Check sheet for the modelled part. Datum: model origin and axes. Units: mm. Face numbers are marked on the shaded views. A direction names the side the tool comes from. Coordinates: 2 decimals unless noted, no trailing zeros. Write each loop counter-clockwise with the first axis right and the second up, starting at its lowest first coordinate (ties: lowest second). Pieces come first, ordered by that corner, then holes. Notation, with made-up numbers: (62.5, -38.5) -> (111.5, -38.5) arc R23 cw to (111.5, -11.5) -> close; hole circle Ø1 at (78.25, 86). An arc over 180 degrees is marked (long way). Put each result on its own line as item: value.
```python
from build123d import *

# Parameters (mm, degrees)
F0_W      = 63.5
F0_H      = 47.625
F1_DEPTH  = 76.2
F2_W      = 41.275
F2_H      = 63.5
F3_DEPTH  = 25.4
F4_R      = 8.255
F6_W      = 12.7
F6_H      = 15.875
F7_DEPTH  = 1.5875
F8_R      = 3.175
F9_W      = 3.175
F9_H      = 6.35
F10_DEPTH = 25.4
F11_R     = 1.58749
F12_W     = 25.4
F12_H     = 47.625
F13_DEPTH = 1.5875
F14_R     = 1.5875


# Not quite as in the source:
# - a fillet or chamfer is up to 0.001 mm smaller than in the source, because OpenCascade refuses the exact size


with BuildPart() as f1:
    # F0 (on Top) → F1 (new body)
    with BuildSketch(Plane.XY):
        Rectangle(F0_W, F0_H)
    extrude(amount=F1_DEPTH)

    # F2 (on face) → F3 (join)
    with BuildSketch(Plane.XZ.offset(23.8125)):
        with Locations((0, 33.3375)):
            Rectangle(F2_W, F2_H)
    extrude(amount=F3_DEPTH)

    # F4
    f4_edges = [f1.edges().sort_by_distance(p)[0] for p in [
        (-20.6375, -36.5125, 65.0875),
        (20.6375, -36.5125, 65.0875),
        (-20.6375, -36.5125, 1.5875),
        (20.6375, -36.5125, 1.5875),
        (20.6375, -49.2125, 33.3375),
        (0, -49.2125, 65.0875),
        (-20.6375, -49.2125, 33.3375),
        (0, -49.2125, 1.5875),
    ]]
    fillet(f4_edges, radius=F4_R)

    # F5: F1 across plane


with BuildPart() as f1_1:
    add(f1.part)
    add(f1.part.mirror(Plane.XZ))

    # F6 (on face) → F7 (join)
    with BuildSketch(Plane(origin=(0, 0, 0), x_dir=(1, 0, 0), z_dir=(0, 0, -1))):
        with Locations((-25.4, 31.75)):
            Rectangle(F6_W, F6_H)
        with Locations((25.4, 31.75)):
            Rectangle(F6_W, F6_H)
        with Locations((25.4, -31.75)):
            Rectangle(F6_W, F6_H)
        with Locations((-25.4, -31.75)):
            Rectangle(F6_W, F6_H)
    extrude(amount=-F7_DEPTH)

    # F8
    f8_edges = [f1_1.edges().sort_by_distance(p)[0] for p in [
        (-31.75, -39.6875, 0.79375),
        (-19.05, -39.6875, 0.79375),
        (19.05, -39.6875, 0.79375),
        (31.75, -39.6875, 0.79375),
        (31.75, 39.6875, 0.79375),
        (19.05, 39.6875, 0.79375),
        (-19.05, 39.6875, 0.79375),
        (-31.75, 39.6875, 0.79375),
    ]]
    fillet(f8_edges, radius=F8_R)

    # F9 (on face) → F10 (cut)
    with BuildSketch(Plane(origin=(0, 0, 0), x_dir=(1, 0, 0), z_dir=(0, 0, -1))):
        with Locations((-25.4, 31.75)):
            Rectangle(F9_W, F9_H)
        with Locations((25.4, 31.75)):
            Rectangle(F9_W, F9_H)
        with Locations((25.4, -31.75)):
            Rectangle(F9_W, F9_H)
        with Locations((-25.4, -31.75)):
            Rectangle(F9_W, F9_H)
    extrude(amount=-F10_DEPTH, mode=Mode.SUBTRACT)

    # F11 (radius 1.5875 in the source; OpenCascade refuses exactly that, so slightly less here)
    f11_edges = [f1_1.edges().sort_by_distance(p)[0] for p in [
        (-26.9875, -34.925, 0.79375),
        (-23.8125, -34.925, 0.79375),
        (-26.9875, -28.575, 0.79375),
        (-23.8125, -28.575, 0.79375),
        (26.9875, -28.575, 0.79375),
        (26.9875, -34.925, 0.79375),
        (23.8125, -34.925, 0.79375),
        (23.8125, -28.575, 0.79375),
        (-26.9875, 34.925, 0.79375),
        (-23.8125, 34.925, 0.79375),
        (-23.8125, 28.575, 0.79375),
        (-26.9875, 28.575, 0.79375),
        (23.8125, 28.575, 0.79375),
        (26.9875, 34.925, 0.79375),
        (23.8125, 34.925, 0.79375),
        (26.9875, 28.575, 0.79375),
    ]]
    fillet(f11_edges, radius=F11_R)

    # F12 (on face) → F13 (join)
    with BuildSketch(Plane.XY.offset(76.2)):
        Rectangle(F12_W, F12_H)
    extrude(amount=F13_DEPTH)

    # F14
    f14_edges = [f1_1.edges().sort_by_distance(p)[0] for p in [
        (0, -23.8125, 77.7875),
        (0, 23.8125, 77.7875),
    ]]
    fillet(f14_edges, radius=F14_R)


solid = f1_1.part
```
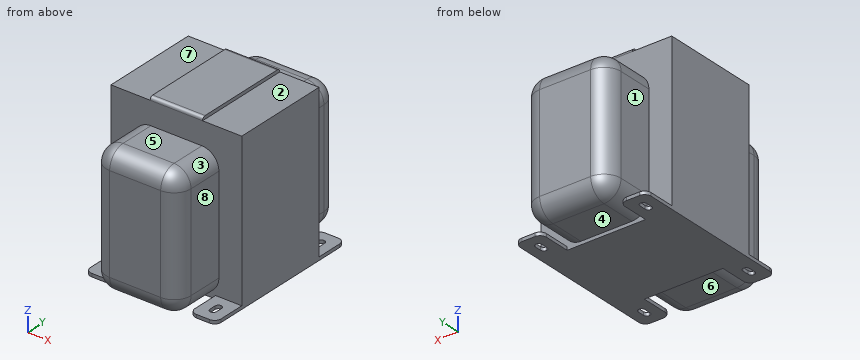
Q1. Material ranges on line 1 along X through (y, z) = (34.5, 10); line 2 along Z through (x, y) = (23.5, 14.5); line 3 along Z through (x, y) = (-21.5, -39), recorded low to high.
Recorded:
line 1: x = -20.64 to 20.64
line 2: z = 0 to 76.2
line 3: z = 0 to 1.59
Q2. Cross-section at A-A (x = 0). Record the cut outline in (y, z) (1 decimal).
Recorded:
outline: (-49.2, 9.8) arc R8.3 ccw to (-41, 1.6) -> (-23.8, 1.6) -> (-23.8, 0) -> (23.8, 0) -> (23.8, 1.6) -> (41, 1.6) arc R8.3 ccw to (49.2, 9.8) -> (49.2, 56.8) arc R8.3 ccw to (41, 65.1) -> (23.8, 65.1) -> (23.8, 76.2) arc R1.6 ccw to (22.2, 77.8) -> (-22.2, 77.8) arc R1.6 ccw to (-23.8, 76.2) -> (-23.8, 65.1) -> (-41, 65.1) arc R8.3 ccw to (-49.2, 56.8) -> close
Q3. Mould release check, pull along X, two halves, no side actions. Record for the marked faces 6, 7 and 8: released by +X, released by -X, zero draft, split by the parting line, or undercut.
Recorded:
face 6: undercut
face 7: zero draft
face 8: released by +X
Q4. Cross-section at D-D (z = 67.5). Record the cut outline in (x, y), plus the area to 3 significant figures.
Recorded:
outline: (-31.75, -23.81) -> (31.75, -23.81) -> (31.75, 23.81) -> (-31.75, 23.81) -> close
area: 3,020 mm2
Q5. Cross-section at C-C (z = 59). Record the cut outline in (x, y).
Recorded:
outline: (-31.75, -23.81) -> (-20.35, -23.81) -> (-20.35, -40.96) arc R7.97 ccw to (-12.38, -48.92) -> (12.38, -48.92) arc R7.97 ccw to (20.35, -40.96) -> (20.35, -23.81) -> (31.75, -23.81) -> (31.75, 23.81) -> (20.35, 23.81) -> (20.35, 40.96) arc R7.97 ccw to (12.38, 48.92) -> (-12.38, 48.92) arc R7.97 ccw to (-20.35, 40.96) -> (-20.35, 23.81) -> (-31.75, 23.81) -> close
Q6. Depth check by flat-ended pin: P1, Ø1.3, axis at y = 2.5, z = 77, coming from the -X side; P2, Ø0.8, axis at x = 25, z = 1, coming from the -Y side; P3, Ø6, axis at x = -24, y = 11.5, coming from the +Z side. Enter the tip coordinate at first touch or a pass-through.
Recorded:
P1: stops at x = -12.7
P2: stops at y = -39.69
P3: stops at z = 76.2
Q7. Tool access check on the marked faces 1, 2, 3, 4 and 5. Record the directions out of +Z, -Z, +X, -X, +Y, -Y that give a thin tool (end or side, any length) a straight path to the whole face; none if there is none.
Recorded:
face 1: +Z, -X, +Y
face 2: +Z, +X, +Y, -Y
face 3: +Z, +X, -Y
face 4: -Z, +Y
face 5: +Z, +X, -X, -Y
